```python
from build123d import *

# Parameters (mm, degrees)
SKETCH1_W           = 8.89
SKETCH1_H           = 5.33
BOSS_EXTRUDE1_DEPTH = 8.38
SKETCH2_W           = 3.81
SKETCH2_H           = 5.33
CUT_EXTRUDE1_DEPTH  = 6.1
SKETCH3_R           = 0.255
BOSS_EXTRUDE2_DEPTH = 6


with BuildPart() as part:
    # Sketch1 → Boss-Extrude1 (new body)
    with BuildSketch(Plane(origin=(0, 0, 0), x_dir=(0, 0, -1), z_dir=(1, 0, 0))):
        with Locations((4.445, 2.665)):
            Rectangle(SKETCH1_W, SKETCH1_H)
    extrude(amount=BOSS_EXTRUDE1_DEPTH)

    # Sketch2 → Cut-Extrude1 (cut)
    with BuildSketch(Plane(origin=(8.38, 0, 0), x_dir=(0, 0, -1), z_dir=(1, 0, 0))):
        with Locations((4.445, 2.665)):
            Rectangle(SKETCH2_W, SKETCH2_H)
    extrude(amount=-CUT_EXTRUDE1_DEPTH, mode=Mode.SUBTRACT)

    # Sketch3 → Boss-Extrude2 (add)
    with BuildSketch(Plane.ZY):
        with Locations((-7.945, 3.935)):
            Circle(SKETCH3_R)
        with Locations((-7.945, 1.395)):
            Circle(SKETCH3_R)
        with Locations((-0.945, 4.57)):
            Circle(SKETCH3_R)
        with Locations((-0.945, 2.665)):
            Circle(SKETCH3_R)
        with Locations((-0.945, 0.76)):
            Circle(SKETCH3_R)
    extrude(amount=BOSS_EXTRUDE2_DEPTH)


solid = part.part
```
Verification items for the finished model (mm, model axes). A direction names the side the tool comes from. Give positions to 0.01 mm unless a question says otherwise; leave off trailing zeros. Write each loop counter-clockwise with the first axis right and the second up, starting at its lowest first coordinate (ties: lowest second). Pieces come first, ordered by that corner, then holes. Notation, with made-up numbers: M 84.25,78.5 L 136.25,78.5 A18 ccw 136.25,108.5 Z; hole C 42.5,79.25 d7. An arc over 180 degrees is marked long. One line per question, with ' | ' between items.
1) Gauge pin test, flat end, axial feed: pin 1 Ø1.6 at (y, z) = (3, -3) entering from -X. Record the tip position at first contact, or that the pin passes through.
Result:
pin 1: stops at x = 0
2) Set-up check for faces 4 (the flat face through (2.28, 3, -4)), 5 (the flat face through (4, 3, -8.89)): record each of +Z, -Z, +X, -X, +Y, -Y from which the full face is reachable in a straight line by a thin tool's end or side.
Result:
face 4: +X, +Y, -Y | face 5: -Z, +X, -X, +Y, -Y
3) Thickness scan on line 1 along Z through (x, y) = (5.75, 0.75); line 2 along Y through (x, z) = (-0.5, -1); line 3 along X through (y, z) = (2.6, -6). Record the ranges inside material, lowest first. Write a range as [from, to].
Result:
line 1: z = [-8.89, -6.35], [-2.54, 0] | line 2: y = [0.51, 1.01], [2.42, 2.91], [4.32, 4.82] | line 3: x = [0, 2.28]
4) Section check D-D on z = -6. Enter the section's corners in (x, y), plus the area to 3 significant figures.
Result:
outline: M 0,0 L 2.28,0 L 2.28,5.33 L 0,5.33 Z | area: 12.2 mm2
5) Section check B-B on y = 4.57. Enter the section's corners in (x, z).
Result:
outline: M -6,-1.2 L 0,-1.2 L 0,-8.89 L 8.38,-8.89 L 8.38,-6.35 L 2.28,-6.35 L 2.28,-2.54 L 8.38,-2.54 L 8.38,0 L 0,0 L 0,-0.69 L -6,-0.69 Z
6) Mould release check, pull along Z, two halves, no side actions. Record for faces 1 (the flat face through (8.38, 3, -8)), 2 (the flat face through (5, 3, -6.35)), 3 (the flat face through (4, 3, 0)): released by +Z, released by -Z, zero draft, split by the parting line, or undercut.
Result:
face 1: zero draft | face 2: undercut | face 3: released by +Z
7) Section check C-C on x = -1.5. Enter the section's corners in (y, z) (3 decimals), plus the area to 3 significant figures.
Result:
outline: C 0.76,-0.945 d0.51; C 1.395,-7.945 d0.51; C 2.665,-0.945 d0.51; C 3.935,-7.945 d0.51; C 4.57,-0.945 d0.51 | area: 1.02 mm2
8) Section check A-A on x = 3. Enter the section's corners in (y, z).
Result:
outline: M 0,-8.89 L 5.33,-8.89 L 5.33,-6.35 L 0,-6.35 Z; M 0,-2.54 L 5.33,-2.54 L 5.33,0 L 0,0 Z
